from build123d import *

# Parameters (mm, degrees)
SKETCH1_W                      = 40
SKETCH1_H                      = 70
BOSS_EXTRUDE1_DEPTH            = 59
SKETCH2_R                      = 11
SKETCH2_R_2                    = 2.5
CUT_EXTRUDE1_DEPTH             = 72.504101247
F_2_5_2_5_DIAMETER_HOLE1_D     = 2.5
F_2_5_2_5_DIAMETER_HOLE1_DEPTH = 7.248924226
F_2_5_2_5_DIAMETER_HOLE1_TIP   = 0.751075774
SKETCH5_W                      = 24
SKETCH5_H                      = 6
CUT_EXTRUDE2_DEPTH             = 3
FILLET2_R                      = 10
FILLET3_R                      = 10
FILLET4_R                      = 10
FILLET5_R                      = 10
SKETCH9_R                      = 3
CUT_EXTRUDE3_DEPTH             = 72.504101247


with BuildPart() as part:
    # Sketch1 → Boss-Extrude1 (new body)
    with BuildSketch(Plane.XY):
        with Locations((0.060830656, 0.062794648)):
            Rectangle(SKETCH1_W, SKETCH1_H)
    extrude(amount=BOSS_EXTRUDE1_DEPTH)

    # Sketch2 → Cut-Extrude1 (cut, through all)
    with BuildSketch(Plane.XY):
        Circle(SKETCH2_R)
        with Locations((-11.313708499, 11.313708499)):
            Circle(SKETCH2_R_2)
        with Locations((-0.122338904, 15.759725587)):
            Circle(SKETCH2_R_2)
        with Locations((11.402693442, 11.263696484)):
            Circle(SKETCH2_R_2)
        with Locations((11.339369089, -11.406422087)):
            Circle(SKETCH2_R_2)
        with Locations((-0.312311964, -16.029099896)):
            Circle(SKETCH2_R_2)
        with Locations((-11.204100775, -11.406422087)):
            Circle(SKETCH2_R_2)
    extrude(amount=CUT_EXTRUDE1_DEPTH, mode=Mode.SUBTRACT)

    # Ø2.5 (2.5) Diameter Hole1
    with Locations(Plane.ZY.offset(19.939169344)):
        with Locations((14.5, 15.062794648), (44.5, 15.062794648), (44.5, -14.937205352), (14.5, -14.937205352)):
            Hole(F_2_5_2_5_DIAMETER_HOLE1_D / 2, depth=F_2_5_2_5_DIAMETER_HOLE1_DEPTH)
            with Locations((0, 0, -(F_2_5_2_5_DIAMETER_HOLE1_DEPTH + F_2_5_2_5_DIAMETER_HOLE1_TIP / 2))):  # 118° drill point
                Cone(0, F_2_5_2_5_DIAMETER_HOLE1_D / 2, F_2_5_2_5_DIAMETER_HOLE1_TIP, mode=Mode.SUBTRACT)

    # Sketch5 → Cut-Extrude2 (cut)
    with BuildSketch(Plane.ZY.offset(19.939169344)):
        with Locations((29.5, -14.937205352)):
            Rectangle(SKETCH5_W, SKETCH5_H)
    extrude(amount=-CUT_EXTRUDE2_DEPTH, mode=Mode.SUBTRACT)

    # Fillet2
    fillet2_edges = [part.edges().sort_by_distance(p)[0] for p in [
        (20.060830656, 35.062794648, 29.5),
    ]]
    fillet(fillet2_edges, radius=FILLET2_R)

    # Fillet3
    fillet3_edges = [part.edges().sort_by_distance(p)[0] for p in [
        (-19.939169344, 35.062794648, 29.5),
    ]]
    fillet(fillet3_edges, radius=FILLET3_R)

    # Fillet4
    fillet4_edges = [part.edges().sort_by_distance(p)[0] for p in [
        (20.060830656, -34.937205352, 29.5),
    ]]
    fillet(fillet4_edges, radius=FILLET4_R)

    # Fillet5
    fillet5_edges = [part.edges().sort_by_distance(p)[0] for p in [
        (-19.939169344, -34.937205352, 29.5),
    ]]
    fillet(fillet5_edges, radius=FILLET5_R)

    # Sketch9 → Cut-Extrude3 (cut, through all)
    with BuildSketch(Plane.XY.offset(59)):
        with Locations((0, 23.01)):
            Circle(SKETCH9_R)
        with Locations((0, -23.01)):
            Circle(SKETCH9_R)
    extrude(amount=-CUT_EXTRUDE3_DEPTH, mode=Mode.SUBTRACT)


solid = part.part
Verification items for the finished model (mm, model axes). A direction names the side the tool comes from. Give positions to 0.01 mm unless a question says otherwise; leave off trailing zeros. Loops run counter-clockwise (first coordinate to the right, second up) from the corner with the lowest first, then second, coordinate; pieces in that order, holes last.
1) Sectioned sample at C-C, the plane x = 8. Enter the section's corners in (y, z), then the cut area to 3 significant figures.
2) Thickness scan on line 1 along X through (y, z) = (0, 19); line 2 along X through (y, z) = (-16, 43.5); line 3 along Y through (x, z) = (-9.5, 52.5). Record the ranges inside material, lowest first.
3) Draft check along X on faces 1 (the cylindrical face through (-0.65, 20.08, 29.91)), 2 (the conical face through (-12.07, -14.87, 44.71)), 3 (the cylindrical face through (17.054, 32.211, 29.913)), 4 (the flat face through (9, -7, 0)). Enter one of: pulls with the +X half, pulls with the -X half, needs draft (parallel to the pull), parting line crosses it, or undercut.
4) Sectioned sample at B-B, the plane x = 0. Enter the section's corners in (y, z), then the cut area to 3 significant figures.
5) Sectioned sample at D-D, the plane z = 51. Count the separate pieces of the cut face and the enclosed holes in it, then the cut area to 3 significant figures.
6) Set-up check for faces 5 (the flat face through (-18, -15, 17.5)), 6 (the cylindrical face through (-10.051, -13.624, 29.087)): record each of +Z, -Z, +X, -X, +Y, -Y from which the full face is reachable in a straight line by a thin tool's end or side.
7) Sectioned sample at A-A, the plane y = 0. Enter the section's corners in (x, z).
8) Depth check by flat-ended pin: pin 1 Ø4 at (x, z) = (12, 23) entering from +Y; pin 2 Ø1.5 at (y, z) = (-14.94, 14.5) entering from -X; pin 3 Ø4 at (x, y) = (-11.31, 11.31) entering from -Z; pin 4 Ø2.5 at (x, z) = (-18.5, 27) entering from +Y. Enter the tip coordinate at first touch or a pass-through.
Answers:
1. outline: (-34.94, 0) - (-7.55, 0) - (-7.55, 59) - (-34.94, 59) - close; (7.55, 0) - (35.06, 0) - (35.06, 59) - (7.55, 59) - close
1. area: 3,240 mm2
2. line 1: x = -19.94 to -11, 11 to 20.06
2. line 2: x = -19.94 to -2.81, 2.19 to 20.06
2. line 3: y = -34.94 to -13.24, -9.58 to -5.55, 5.55 to 9.59, 13.03 to 35.06
3. face 1: undercut
3. face 2: pulls with the -X half
3. face 3: pulls with the +X half
3. face 4: needs draft
4. outline: (-34.94, 0) - (-26.01, 0) - (-26.01, 59) - (-34.94, 59) - close; (-20.01, 0) - (-18.51, 0) - (-18.51, 59) - (-20.01, 59) - close; (-13.55, 0) - (-11, 0) - (-11, 59) - (-13.55, 59) - close; (11, 0) - (13.26, 0) - (13.26, 59) - (11, 59) - close; (18.26, 0) - (20.01, 0) - (20.01, 59) - (18.26, 59) - close; (26.01, 0) - (35.06, 0) - (35.06, 59) - (26.01, 59) - close
4. area: 1,540 mm2
5. separate pieces: 1
5. enclosed holes: 9
5. area: 2,160 mm2
6. face 5: -X
6. face 6: +Z, -Z
7. outline: (-19.94, 0) - (-11, 0) - (-11, 59) - (-19.94, 59) - close; (11, 0) - (20.06, 0) - (20.06, 59) - (11, 59) - close
8. pin 1: stops at y = 35.06
8. pin 2: stops at x = -12.39
8. pin 3: passes through
8. pin 4: stops at y = 31.89
